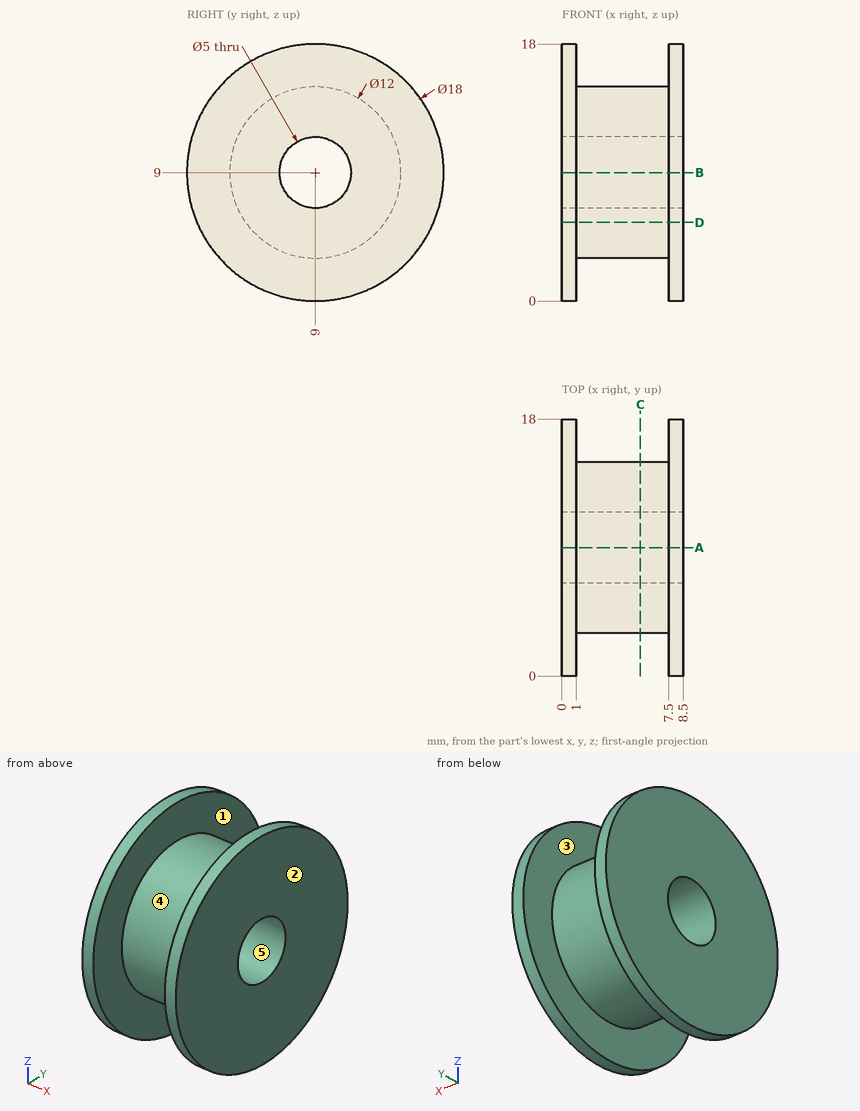
Input: dimensioned drawing with shaded views. Units: mm. Origin: part minimum x, y, z. A direction names the side the tool comes from. Round coordinates to 2 decimals unless told otherwise and drop trailing zeros. Loops run counter-clockwise (first coordinate to the right, second up) from the corner with the lowest first, then second, coordinate; pieces in that order, holes last. Notation, with made-up numbers: M 74.25,-25.5 L 123.25,-25.5 A23 ccw 123.25,-4.5 Z; hole C 78,80 d6. An arc over 180 degrees is marked long. Return JSON: item names as keys, results as strings. Group by question number.
1. Section query C-C on x = 5.5. Output: boundary loops of the cut face in (y, z).
2. Material intervals for line 1 along Z through (x, y) = (3.75, 9); line 2 along X through (y, z) = (15.5, 12.25); line 3 along Y through (x, z) = (8.25, 10.75), sorted ascending. Write a range as from..to.
3. Section query D-D on z = 5.5. Output: boundary loops of the cut face in (x, y).
4. Mould query, pull axis Y, two halves, no side actions, for the marked faces 3, 4 and 5. Classes: released by +Y, released by -Y, zero draft, split by the parting line, or undercut.
5. Pin query (flat end, axial travel): pin 1 (3 mm diameter, centred on x = 3, z = 8.5, fed in from -Y); pin 2 (3 mm diameter, centred on x = 6.5, z = 6, fed in from +Y); pin 3 (1 mm diameter, centred on x = 1, z = 15, fed in from -Y). Return the tip coordinate at first contact, or that it passes through.
6. Reachability of the marked faces 1 and 2 from +Z, -Z, +X, -X, +Y, -Y: full face, straight path, thin tool, end or side. Return the list, or none.
7. Section query A-A on y = 9. Output: boundary loops of the cut face in (x, z), and give its area (3 significant figures).
Checks:
{
 "1": {"outline": "C 9,9 d12; hole C 9,9 d5"},
 "2": {"line 1": "z = 3..6.5, 11.5..15", "line 2": "x = 0..1, 7.5..8.5", "line 3": "y = 0.17..7.21, 10.79..17.83"},
 "3": {"outline": "M 0,0.71 L 1,0.71 L 1,4.13 L 7.5,4.13 L 7.5,0.71 L 8.5,0.71 L 8.5,17.29 L 7.5,17.29 L 7.5,13.87 L 1,13.87 L 1,17.29 L 0,17.29 Z"},
 "4": {"face 3": "zero draft", "face 4": "split by the parting line", "face 5": "undercut"},
 "5": {"pin 1": "stops at y = 3", "pin 2": "stops at y = 17.8", "pin 3": "stops at y = 1.88"},
 "6": {"face 1": "none", "face 2": "+Z, -Z, +X, +Y, -Y"},
 "7": {"outline": "M 0,0 L 1,0 L 1,3 L 7.5,3 L 7.5,0 L 8.5,0 L 8.5,6.5 L 0,6.5 Z; M 0,11.5 L 8.5,11.5 L 8.5,18 L 7.5,18 L 7.5,15 L 1,15 L 1,18 L 0,18 Z", "area": "71.5 mm²"}
}
